from build123d import *

# Parameters (mm, degrees)
F0_R     = 85.09
F1_DEPTH = 4.7625
F2_R     = 75.803125
F3_DEPTH = 4.7625
F4_SIZE  = 1.5875


with BuildPart() as f1:
    # F0 (on Front) → F1 (new body)
    with BuildSketch(Plane.XZ):
        Circle(F0_R)
    extrude(amount=F1_DEPTH)

    # F2 (on face) → F3 (cut)
    with BuildSketch(Plane.XZ.offset(4.7625)):
        Circle(F2_R)
    extrude(amount=-F3_DEPTH, mode=Mode.SUBTRACT)

    # F4
    f4_edges = [f1.edges().sort_by_distance(p)[0] for p in [
        (-85.09, -4.7625, 0),
    ]]
    chamfer(f4_edges, length=F4_SIZE)


solid = f1.part
Input: part model. Units: mm. Frame: model coordinates. Give positions to 0.01 mm unless a question says otherwise; leave off trailing zeros. Write each loop counter-clockwise with the first axis right and the second up, starting at its lowest first coordinate (ties: lowest second). Pieces come first, ordered by that corner, then holes. Notation, with made-up numbers: M 12.25,7 L 71.25,7 A19 ccw 71.25,34 Z; hole C 88.25,-39 d7. An arc over 180 degrees is marked long. Use one line per item in the form item = value.
1. First-contact query: P1, Ø12, axis at x = -64, z = 7, coming from the -Y side; P2, Ø1, axis at y = -2.5, z = -35, coming from the -X side; P3, Ø10, axis at x = -66, z = -44, coming from the +Y side. Flat tips, straight axial feed; report the tip coordinate or a pass-through.
Outcome:
P1 = through
P2 = -77.78
P3 = 0
2. Mould query, pull axis X, two halves, no side actions, for faces 1 (the face through (-67.52, -1.57, -51.78)), 2 (the face through (18, -4.762, -74)), 3 (the face through (-60.15, -2.41, -46.13)). Classes: released by +X, released by -X, zero draft, split by the parting line, or undercut.
Outcome:
face_1 = split by the parting line
face_2 = zero draft
face_3 = undercut
3. Ray query, L1, parallel to Z at x = 0, y = -3.2 (3 decimals); L2, parallel to Z at x = 44.5, y = -3.55; L3, parallel to X at y = -1.3, z = 51. Return the intervals inside material, ascending.
Outcome:
L1 = -85.065 to -75.803, 75.803 to 85.065
L2 = -72.09 to -61.37, 61.37 to 72.09
L3 = -68.11 to -56.08, 56.08 to 68.11
4. Cut plane B-B on z = 0. Return loops of the section in (x, y) (1 decimal).
Outcome:
outline = M -85.1,-3.2 L -83.5,-4.8 L -75.8,-4.8 L -75.8,0 L -85.1,0 Z; M 75.8,-4.8 L 83.5,-4.8 L 85.1,-3.2 L 85.1,0 L 75.8,0 Z
5. Cut plane C-C on y = -1.7. Return loops of the section in (x, z).
Outcome:
outline = C 0,0 d170.18; hole C 0,0 d151.61
6. Cut plane A-A on x = 0. Return loops of the section in (y, z) (1 decimal), and give its area (3 significant figures).
Outcome:
outline = M -4.8,-83.5 L -3.2,-85.1 L 0,-85.1 L 0,-75.8 L -4.8,-75.8 Z; M -4.8,75.8 L 0,75.8 L 0,85.1 L -3.2,85.1 L -4.8,83.5 Z
area = 85.9 mm²
